Can you work these out from the model? Positions are in its coordinate system, mm. Face numbers are marked on the shaded views. A direction names the side the tool comes from. Round coordinates to 2 decimals unless told otherwise and drop trailing zeros. Order: outer loops, then holes, each group sorted by start corner. A loop starts at its lowest first (then second) coordinate and runs counter-clockwise, first axis right, second up.
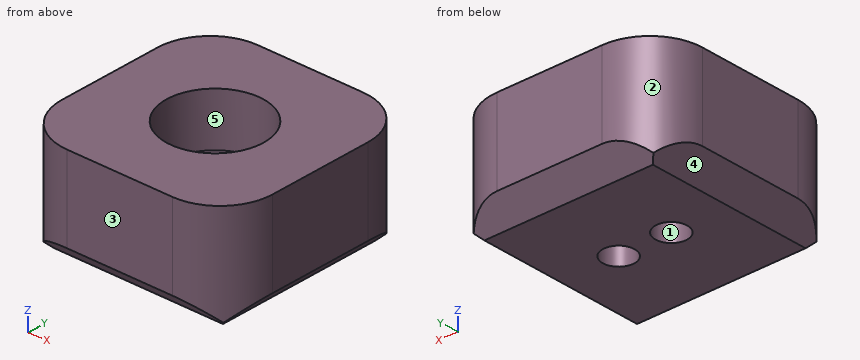
Autodesk Inventor part; units mm, degrees
ref_plane "YZ Plane" through (0, 0, 0) normal (1, 0, 0) x (0, 1, 0)
ref_plane "XZ Plane" through (0, 0, 0) normal (0, 1, 0) x (-1, 0, 0)
ref_plane "XY Plane" through (0, 0, 0) normal (0, 0, 1) x (1, 0, 0)
sketch "Sketch1" plane through (0, 0, 0) normal (0, 0, 1) x (1, 0, 0)
  line L0 (0, 0) -> (12.7, 0)
  line L1 (12.7, 0) -> (12.7, 12.7)
  line L2 (12.7, 12.7) -> (0, 12.7)
  line L3 (0, 12.7) -> (0, 0)
  dimension "d0" = 12.7
  dimension "d1" = 12.7
extrude "Extrusion1" add sketch "Sketch1" along normal blind 6.35
sketch "Sketch2" plane through (0, 0, 6.35) normal (0, 0, 1) x (1, 0, 0)
  line L0 (12.7, 12.7) -> (0, 12.7) construction
  line L1 (0, 0) -> (12.7, 0) construction
  line L2 (0, 12.7) -> (12.7, 0) construction
  line L3 (0, 0) -> (12.7, 12.7) construction
  circle A0 centre (6.35, 6.35) radius 2.921
  dimension "d4" = 5.842
extrude "Extrusion2" cut sketch "Sketch2" against normal blind 3.175
sketch "Sketch3" plane through (6.35, 6.35, 3.175) normal (0, 0, 1) x (1, 0, 0)
  circle A0 centre (0, 0) radius 2.921 construction
  line L0 (-6.35, 0) -> (6.35, 0) construction
  line L1 (-6.35, 6.35) -> (-6.35, -6.35) construction
  line L2 (6.35, -6.35) -> (6.35, 6.35) construction
  circle A1 centre (-1.5875, 0) radius 0.635 construction
  circle A2 centre (1.5875, 0) radius 0.635 construction
  line L3 (-0.9525, 6.35) -> (-0.9525, -6.35) construction
  line L4 (0.9525, -6.35) -> (0.9525, 6.35) construction
  point P0 (1.5875, 0)
  dimension "d7" = 1.27
  dimension "d8" = 1.27
  dimension "d9" = 1.5875
  dimension "d10" = 1.5875
  dimension "d11" = 1.905
  dimension "d26" = 3.175
hole "Hole1" at (4.7625, 6.35, 3.175) at (7.9375, 6.35, 3.175) direction (0, 0, -1) diameter 1.905 end through all
chamfer "Chamfer2" distance 1.27 angle 45 4 edges at (6.35, 0, 0) (12.7, 6.35, 0) (6.35, 12.7, 0) (0, 6.35, 0)
fillet "Fillet1" radius 3.175 4 edges at (12.7, 0, 3.81) (12.7, 12.7, 3.81) (0, 12.7, 3.81) (0, 0, 3.81)
equation "\"d10\" = d9"
properties part number "testled"
(1) On a 3-axis mill with a long thin cutter (end or side, diameter ignored), from which of +Z, -Z, +X, -X, +Y, -Y can I reach the whole of each face in a straight line? I mean the marked faces 4 and 5. Say none if no direction works.
(2) I want a section at D-D, the plane x = 6.35. List the corners of the cut face in (y, z) for me (3 decimals), plus the area to 3 significant figures.
(3) If we mould it in two halves opening along X, with no side actions, what happens to the marked faces 1, 2 and 3? For each: pulls with the +X half, pulls with the -X half, needs draft (parallel to the pull), parting line crosses it, or undercut.
(4) I want a section at B-B, the plane z = 4.5. List the corners of the cut face in (x, y) for me (3 decimals), plus the area to 3 significant figures.
(5) I'm going to push flat-ended pins straight in: pin 1 Ø1 at (x, y) = (10.5, 3) entering from -Z; pin 2 Ø4.5 at (x, y) = (6.35, 6.35) entering from +Z (3 decimals). Where does each tip first touch, or does it pass through?
(6) Please list where these lines run through material, in increasing order: probe 1 along X at (y, z) = (6.35, 1.5) (3 decimals); probe 2 along X at (y, z) = (6.75, 2.5); probe 3 along Y at (x, z) = (6.35, 4).
(7) I want a section at C-C, the plane z = 1. Give the number of separate pieces and of enclosed holes in the cut face, plus the area to 3 significant figures.
(8) I want a section at A-A, the plane y = 6.35. List the corners of the cut face in (x, z) for me (3 decimals), plus the area to 3 significant figures.
Ans:
1. face 4: -Z, -X, +Y, -Y
1. face 5: +Z
2. outline: (0, 1.27) - (1.27, 0) - (11.43, 0) - (12.7, 1.27) - (12.7, 6.35) - (9.271, 6.35) - (9.271, 3.175) - (3.429, 3.175) - (3.429, 6.35) - (0, 6.35) - close
2. area: 60.5 mm2
3. face 1: undercut
3. face 2: pulls with the -X half
3. face 3: needs draft
4. outline: (0, 3.175) arc R3.175 ccw to (3.175, 0) - (9.525, 0) arc R3.175 ccw to (12.7, 3.175) - (12.7, 9.525) arc R3.175 ccw to (9.525, 12.7) - (3.175, 12.7) arc R3.175 ccw to (0, 9.525) - close; hole circle Ø5.842 at (6.35, 6.35)
4. area: 126 mm2
5. pin 1: stops at z = 0
5. pin 2: stops at z = 3.175
6. probe 1: x = 0 to 3.81, 5.715 to 6.985, 8.89 to 12.7
6. probe 2: x = 0 to 3.9, 5.63 to 7.07, 8.8 to 12.7
6. probe 3: y = 0 to 3.43, 9.27 to 12.7
7. separate pieces: 1
7. enclosed holes: 2
7. area: 138 mm2
8. outline: (0, 1.27) - (1.27, 0) - (3.81, 0) - (3.81, 3.175) - (3.429, 3.175) - (3.429, 6.35) - (0, 6.35) - close; (5.715, 0) - (6.985, 0) - (6.985, 3.175) - (5.715, 3.175) - close; (8.89, 0) - (11.43, 0) - (12.7, 1.27) - (12.7, 6.35) - (9.271, 6.35) - (9.271, 3.175) - (8.89, 3.175) - close
8. area: 48.4 mm2
